Design review of the part built by this model. Coordinates are the model's own, in mm. Give positions to 0.01 mm unless a question says otherwise; leave off trailing zeros. Order: outer loops, then holes, each group sorted by start corner. A loop starts at its lowest first (then second) coordinate and runs counter-clockwise, first axis right, second up. Notation, with made-up numbers: (-25.75, 2) -> (27.25, 2) arc R14 ccw to (27.25, 15) -> close; hole circle Ø3 at (81.25, -18.5). An arc over 180 degrees is marked (long way). Use a Markdown table: item, result. Add a question column.
```python
from build123d import *

# Parameters (mm, degrees)
SKETCH1_W           = 50
SKETCH1_H           = 22.5
BOSS_EXTRUDE1_DEPTH = 2
SKETCH2_R           = 8.25
CUT_EXTRUDE1_DEPTH  = 2
SKETCH3_W           = 50
SKETCH3_H           = 2
BOSS_EXTRUDE2_DEPTH = 2


with BuildPart() as part:
    # Sketch1 → Boss-Extrude1 (new body)
    with BuildSketch(Plane.XY):
        with Locations((25, 11.25)):
            Rectangle(SKETCH1_W, SKETCH1_H)
    extrude(amount=BOSS_EXTRUDE1_DEPTH)

    # Sketch2 → Cut-Extrude1 (cut)
    with BuildSketch(Plane.XY.offset(2)):
        with Locations((11.75, 13.75)):
            Circle(SKETCH2_R)
        with Locations((38.25, 13.75)):
            Circle(SKETCH2_R)
    extrude(amount=-CUT_EXTRUDE1_DEPTH, mode=Mode.SUBTRACT)

    # Sketch3 → Boss-Extrude2 (add)
    with BuildSketch(Plane(origin=(0, 22.5, 0), x_dir=(1, 0, 0), z_dir=(0, 1, 0))):
        with Locations((25, -1)):
            Rectangle(SKETCH3_W, SKETCH3_H)
    extrude(amount=BOSS_EXTRUDE2_DEPTH)


solid = part.part
```
1) Add section A-A (y = 13.75). Give the boundary of the cut face in (x, z), then the cut area to 3 significant figures.
2) For L1, parallel to Y at x = 38.25, z = 0.5; L2, parallel to X at y = 14.5, z = 1; L3, parallel to X at y = 16.75, z = 1.55, list the stretches that pass through material, from the lowest coordinate up. Write a range as [from, to].
3) Add section C-C (z = 1). Give the boundary of the cut face in (x, y), then the cut area to 3 significant figures.
4) Add section B-B (x = 11.75). Give the boundary of the cut face in (y, z), then the cut area to 3 significant figures.
5) Add section D-D (y = 6). Give the boundary of the cut face in (x, z).
6) The part is to be moulded in two halves that separate along X. For faces 1 (the cylindrical face through (19.62, 16.23, 1.01)), 2 (the flat face through (50, 12, 1)), 3 (the flat face through (25, 24.5, 1)), 4 (the flat face through (0, 12, 1)), say which applies: +X half, -X half, draft (parallel to the pull), parting line (faces both ways), or undercut.
Worked answers:
| question | item | result |
|---|---|---|
| 1 | outline | (0, 0) -> (3.5, 0) -> (3.5, 2) -> (0, 2) -> close; (20, 0) -> (30, 0) -> (30, 2) -> (20, 2) -> close; (46.5, 0) -> (50, 0) -> (50, 2) -> (46.5, 2) -> close |
| 1 | area | 34.0 mm^2 |
| 2 | L1 | [0, 5.5], [22, 24.5] |
| 2 | L2 | [0, 3.53], [19.97, 30.03], [46.47, 50] |
| 2 | L3 | [0, 4.06], [19.44, 30.56], [45.94, 50] |
| 3 | outline | (0, 0) -> (50, 0) -> (50, 24.5) -> (0, 24.5) -> close; hole circle Ø16.5 at (11.75, 13.75); hole circle Ø16.5 at (38.25, 13.75) |
| 3 | area | 797 mm^2 |
| 4 | outline | (0, 0) -> (5.5, 0) -> (5.5, 2) -> (0, 2) -> close; (22, 0) -> (24.5, 0) -> (24.5, 2) -> (22, 2) -> close |
| 4 | area | 16.0 mm^2 |
| 5 | outline | (0, 0) -> (8.92, 0) -> (8.92, 2) -> (0, 2) -> close; (14.58, 0) -> (35.42, 0) -> (35.42, 2) -> (14.58, 2) -> close; (41.08, 0) -> (50, 0) -> (50, 2) -> (41.08, 2) -> close |
| 6 | face 1 | undercut |
| 6 | face 2 | +X half |
| 6 | face 3 | draft |
| 6 | face 4 | -X half |
